from build123d import *

# Parameters (mm, degrees)
F0_W        = 23.6010048538
F0_H        = 117.7456714213
F1_DEPTH    = 2.032
F2_R        = 5.08
F3_W        = 23.3416529372
F3_H        = 43.9601168036
F4_DEPTH    = 2.032
F5_T1_DEPTH = 43.6616529372


# Not quite as in the source:
# - a fillet or chamfer that OpenCascade refuses, or shapes differently, is made with other operations: its cross-section is extruded or revolved along the edge and cut away or added


with BuildPart() as f1:
    # F0 (on Front) → F1 (new body)
    with BuildSketch(Plane.XZ):
        with Locations((-1.9451379776, -11.8005033582)):
            Rectangle(F0_W, F0_H)
    extrude(amount=-F1_DEPTH)

    # F2
    f2_edges = [f1.edges().sort_by_distance(p)[0] for p in [
        (-13.74564, 1.016, 47.072332),
        (9.855364, 1.016, 47.072332),
        (9.855364, 1.016, -70.673339),
        (-13.74564, 1.016, -70.673339),
    ]]
    fillet(f2_edges, radius=F2_R)

    # F3 (on face) → F4 (join)
    with BuildSketch(Plane(origin=(0, 0, -70.6733390689), x_dir=(1, 0, 0), z_dir=(0, 0, -1))):
        with Locations((-2.3341649212, 21.9800584018)):
            Rectangle(F3_W, F3_H)
    extrude(amount=-F4_DEPTH)

    # F5: fillet of radius 5.08 on 1 edges, made by hand

    # F5_s2 → F5_t1 (cut)
    with BuildSketch(Plane.YZ.offset(-24.1649913898)):
        with BuildLine():
            ThreePointArc((-39.8961168036, -70.6733390689), (-42.1679618688, -70.1370291992), (-43.9601168036, -68.6413390689))
            Line((-43.9601168036, -68.6413390689), (-43.9601168036, -70.6733390689))
            Line((-43.9601168036, -70.6733390689), (-39.8961168036, -70.6733390689))
        make_face()
    extrude(amount=F5_T1_DEPTH, mode=Mode.SUBTRACT)


solid = f1.part
Geometry: final body of the model. Coordinates: model frame, mm. A direction names the side the tool comes from. Give positions to 0.01 mm unless a question says otherwise; leave off trailing zeros. Loops run counter-clockwise (first coordinate to the right, second up) from the corner with the lowest first, then second, coordinate; pieces in that order, holes last. Notation, with made-up numbers: (83, 24) -> (88, 24) arc R19 ccw to (88, 37) -> close; hole circle Ø7 at (48, -4.5). An arc over 180 degrees is marked (long way). Put each result on its own line as item: value.
1. Cut plane C-C (y = -20.5). Return the cut outline in (x, z) (3 decimals).
Taken from the geometry:
outline: (-14.005, -70.673) -> (9.337, -70.673) -> (9.337, -68.641) -> (-14.005, -68.641) -> close
2. Pin query (flat end, axial travel): P1, Ø4, axis at x = 5.5, y = -30, coming from the +Z side; P2, Ø5, axis at x = 3, z = -12, coming from the -Y side; P3, Ø1.6, axis at y = -28.5, z = -70, coming from the +X side. Return the tip coordinate at first contact, or that it passes through.
Taken from the geometry:
P1: stops at z = -68.64
P2: stops at y = 0
P3: stops at x = 9.34
3. Ray query, line 1 along Z through (x, y) = (6.25, -21); line 2 along Y through (x, z) = (6.75, 30.5). Return the intervals inside material, ascending. Write a range as [from, to].
Taken from the geometry:
line 1: z = [-70.67, -68.64]
line 2: y = [0, 2.03]
4. Cut plane A-A (x = -3.75). Return the cut outline in (y, z), plus the area to 3 significant figures.
Taken from the geometry:
outline: (-43.96, -68.64) arc R5.08 ccw to (-39.9, -70.67) -> (2.03, -70.67) -> (2.03, 47.07) -> (0, 47.07) -> (0, -68.64) -> close
area: 326 mm2
5. Set-up query: faces 1 (the cylindrical face through (8.33, 1.03, -69.22)), 2 (the flat face through (-2, 0, -10)), 3 (the cylindrical face through (-12.297, 1.03, -69.146)). Return all of +Z, -Z, +X, -X, +Y, -Y with unobstructed straight access to the full face (end or side cutting, diameter ignored); none if empty.
Taken from the geometry:
face 1: -Z, +X, +Y
face 2: +Z, +X, -X, -Y
face 3: -Z, -X, +Y
6. Cut plane D-D (x = -11). Return the cut outline in (y, z), plus the area to 3 significant figures.
Taken from the geometry:
outline: (-43.96, -68.64) arc R5.08 ccw to (-39.9, -70.67) -> (0, -70.67) -> (0, -70.11) -> (2.03, -70.11) -> (2.03, 46.5) -> (0, 46.5) -> (0, -68.64) -> close
area: 324 mm2
7. Cut plane B-B (z = -7). Return the cut outline in (x, y), plus the area to 3 significant figures.
Taken from the geometry:
outline: (-13.75, 0) -> (9.86, 0) -> (9.86, 2.03) -> (-13.75, 2.03) -> close
area: 48.0 mm2
